Here's how the part is built. I have some questions about the finished solid (model axes, mm). Face numbers are marked on the shaded views. A direction names the side the tool comes from. Coordinates: 2 decimals unless noted, no trailing zeros. Write each loop counter-clockwise with the first axis right and the second up, starting at its lowest first coordinate (ties: lowest second). Pieces come first, ordered by that corner, then holes.
(1) For pin 1 Ø2 at (x, y) = (2, 4) entering from +Z; pin 2 Ø1 at (y, z) = (4.5, -5) entering from -X; pin 3 Ø2 at (x, y) = (-17.5, 4) entering from +Z, each with a flat end and sliding along its axis, tell me the tip position at first contact or that it passes through.
(2) Please list where these lines run through material, in increasing order: probe 1 along Z at (x, y) = (2.5, 2.75); probe 2 along X at (y, z) = (5.5, -7); probe 3 along X at (y, z) = (2.75, 0).
(3) Imagine slicing it at D-D, the plane x = -2. List the corners of the cut face in (y, z) for me, plus the area to 3 significant figures.
(4) Imagine slicing it at B-B, the plane y = 1.25. List the corners of the cut face in (x, z) for me.
(5) Thinking about a two-plate mould opening in X: for the marked faces 4, 5, 6 and 7, which applies, released by +X, released by -X, zero draft, split by the parting line, or undercut?
(6) Imagine slicing it at A-A, the plane x = 2.5. List the corners of the cut face in (y, z) for me.
(7) Which directions (+Z, -Z, +X, -X, +Y, -Y) give clear straight access to the entire face, cutting with the end or side of a thin tool? Please do the marked faces 1, 2 and 3.
(8) Imagine slicing it at C-C, the plane z = 1.75. List the corners of the cut face in (x, y) for me.
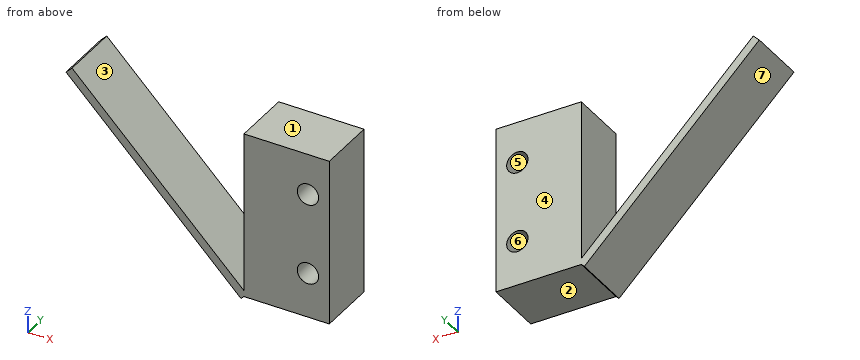
Autodesk Inventor part; units mm, degrees
ref_plane "РабПлоскость1" through (-5, 0, -9.8) normal (-0.7071, 0, -0.7071) x (0, 1, 0)
ref_plane "YZ Plane" through (0, 0, 0) normal (1, 0, 0) x (0, 1, 0)
ref_plane "XZ Plane" through (0, 0, 0) normal (0, 1, 0) x (-1, 0, 0)
sketch "Эскиз1" plane through (0, 0, 0) normal (0, 1, 0) x (-1, 0, 0)
  line L0 (5, -9.8) -> (-5, -9.8)
  line L1 (-5, -9.8) -> (-5, 9.8)
  line L2 (-5, 9.8) -> (5, 9.8)
  line L3 (5, 9.8) -> (5, -9.8)
  line L4 (5, -9.8) -> (-5, 9.8) construction
  line L5 (-5, -9.8) -> (5, 9.8) construction
  point P0 (0, 0)
  dimension "d0" = 10
  dimension "d1" = 19.6
extrude "Выдавливание1" add sketch "Эскиз1" along normal blind 6.9
sketch "Эскиз2" plane through (0, 6.9, 0) normal (0, 1, 0) x (1, 0, 0)
  circle A0 centre (2.5, -4.9766) radius 1.25
  circle A1 centre (2.5, 4.5234) radius 1.25
  line L0 (5, -9.8) -> (5, 9.8)
  line L1 (2.5, -4.9766) -> (2.5, -0.2266)
  line L2 (2.5, -0.2266) -> (2.5, 4.5234)
  point P0 (0, 0)
  dimension "d4" = 2.5
  dimension "d5" = 2.5
  dimension "d6" = 9.5
  dimension "d7" = 2.5
  dimension "d8" = 2.5
extrude "Выдавливание2" cut sketch "Эскиз2" against normal blind 6.9
ref_plane "РабПлоскость1" through (-5, 0, -9.8) normal (-0.7071, 0, -0.7071) x (0, 1, 0)
sketch "Эскиз3" plane through (-5, 0, -9.8) normal (-0.7071, 0, -0.7071) x (0, 1, 0)
  line L0 (0, 0) -> (6.9, 0)
  line L1 (0, 0) -> (6.9, 0)
  line L2 (6.9, 0) -> (6.9, -29)
  line L3 (6.9, -29) -> (0, -29)
  line L4 (0, -29) -> (0, 0)
  point P0 (0, -3.3941)
  dimension "d12" = 6.9
  dimension "d13" = 29
extrude "Выдавливание3" add sketch "Эскиз3" along normal mid plane 1
properties part number "концевик"
Recorded:
1. pin 1: stops at z = 9.8
1. pin 2: stops at x = -11.01
1. pin 3: stops at z = 4.41
2. probe 1: z = -9.8 to -5.77, -3.27 to 3.73, 6.23 to 9.8
2. probe 2: x = -8.51 to -7.09, -5 to 5
2. probe 3: x = -15.51 to -14.09, -5 to 5
3. outline: (0, -9.8) - (6.9, -9.8) - (6.9, 9.8) - (0, 9.8) - close
3. area: 135 mm2
4. outline: (-25.86, 10.35) - (-5.35, -10.15) - (-5, -9.8) - (5, -9.8) - (5, 9.8) - (-5, 9.8) - (-5, -9.09) - (-25.15, 11.06) - close; hole circle Ø2.5 at (2.5, -4.52); hole circle Ø2.5 at (2.5, 4.98)
5. face 4: zero draft
5. face 5: undercut
5. face 6: undercut
5. face 7: released by -X
6. outline: (0, -9.8) - (6.9, -9.8) - (6.9, -5.77) - (0, -5.77) - close; (0, -3.27) - (6.9, -3.27) - (6.9, 3.73) - (0, 3.73) - close; (0, 6.23) - (6.9, 6.23) - (6.9, 9.8) - (0, 9.8) - close
7. face 1: +Z, +X, +Y, -Y
7. face 2: -Z, +X, +Y, -Y
7. face 3: +Z, +Y, -Y
8. outline: (-17.26, 0) - (-15.84, 0) - (-15.84, 6.9) - (-17.26, 6.9) - close; (-5, 0) - (5, 0) - (5, 6.9) - (-5, 6.9) - close
